Design review of the part built by this model. Coordinates are the model's own, in mm. Face numbers are marked on the shaded views. A direction names the side the tool comes from. Coordinates: 2 decimals unless noted, no trailing zeros. Put each result on its own line as item: value. Start each with the question number.
(1) For probe 1 along Z at (x, y) = (0.05, 0); probe 2 along X at (y, z) = (-3.25, 6) (3 decimals); probe 3 along Y at (x, z) = (1.85, -6), list the stretches that pass through material, from the lowest coordinate up. Write a range as [from, to].
(2) The part is to be moulded in two halves that separate along Z. For the marked faces 3 and 4, say which applies: +Z half, -Z half, draft (parallel to the pull), parting line (faces both ways), or undercut.
(3) Clearance check with flat-ended pins moving along their axes: pin 1 (7 mm diameter, centred on y = 0, z = 1.5, fed in from -X) (3 decimals); pin 2 (1.5 mm diameter, centred on x = 1, y = -1.5, fed in from +Z). State where each tip first meets the part, or that it passes through.
(4) For the marked faces 1 and 2, list the 3-axis set-ups (+Z, -Z, +X, -X, +Y, -Y) from which the entire face can be reached by the end or side of a thin tool; tool diameter is ignored.
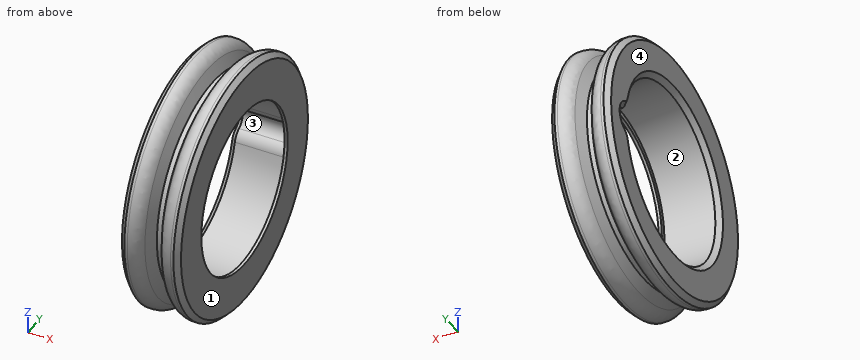
Autodesk Inventor part; units mm, degrees
ref_plane "YZ Plane" through (0, 0, 0) normal (1, 0, 0) x (0, 1, 0)
ref_plane "XZ Plane" through (0, 0, 0) normal (0, 1, 0) x (-1, 0, 0)
ref_plane "XY Plane" through (0, 0, 0) normal (0, 0, 1) x (1, 0, 0)
sketch "Эскиз1" plane through (0, 0, 0) normal (0, 0, 1) x (1, 0, 0)
  line L0 (-2.375, 10.1) -> (-1, 10.1)
  line L1 (2.375, 10.1) -> (2.375, 6.6)
  line L2 (2.125, 7) -> (-2.375, 7)
  line L3 (-2.375, 7) -> (-2.375, 10.1)
  line L4 (-3.325, 0) -> (3.325, 0) construction
  line L5 (0, -2.02) -> (0, 12.12) construction
  line L6 (1, 10.1) -> (2.375, 10.1)
  line L7 (-1, 10.1) -> (-0.2, 8.5)
  line L8 (-0.2, 8.5) -> (0.2, 8.5)
  line L9 (0.2, 8.5) -> (1, 10.1)
  line L10 (2.125, 7) -> (2.125, 6.6)
  line L11 (2.125, 6.6) -> (2.375, 6.6)
  point P0 (0, 0)
  point P1 (0, 8.5)
  dimension "d0" = 7
  dimension "d5" = 0.4
  dimension "d6" = 1.5
  dimension "d7" = 2
  dimension "d12" = 0.25
  dimension "d13" = 3.5
  dimension "d14" = 0.4
  dimension "d16" = 4.5
revolve "Вращение1" add sketch "Эскиз1" angle 360 about axis through (-10, 0, 0) along (1, 0, 0)
sketch "Эскиз2" plane through (-2.375, 0, 0) normal (-1, 0, 0) x (0, 0, 1)
  circle A0 centre (0, 0) radius 7 construction
  circle A1 centre (0, 7) radius 1
  line L0 (0, -14.14) -> (0, 14.14) construction
  dimension "d21" = 2
extrude "Выдавливание1" cut sketch "Эскиз2" against normal up to surface (4.5 mm away)
fillet "Сопряжение1" radius 1.2 4 edges at (-1, -10.1, 0) (1, -10.1, 0) (-0.125, 6.9286, -0.9974) (-0.125, 6.9286, 0.9974)
chamfer "Фаска2" distance 0.4 angle 45 6 edges at (2.375, -10.1, 0) (-2.375, -10.1, 0) (-2.375, -7, 0) (-2.375, 7.0258, 1.2241) (-2.375, 7.0258, -1.2241) (-2.375, 8, 0)
properties part number "Шкив рычага"
Computed values:
1. probe 1: z = [-8.5, -7], [7, 8.5]
1. probe 2: x = [2.125, 2.375]
1. probe 3: y = [-8.12, -3.61], [3.61, 8.12]
2. face 3: undercut
2. face 4: draft
3. pin 1: passes through
3. pin 2: stops at z = 10.04
4. face 1: +Z, -Z, +X, +Y, -Y
4. face 2: -X
